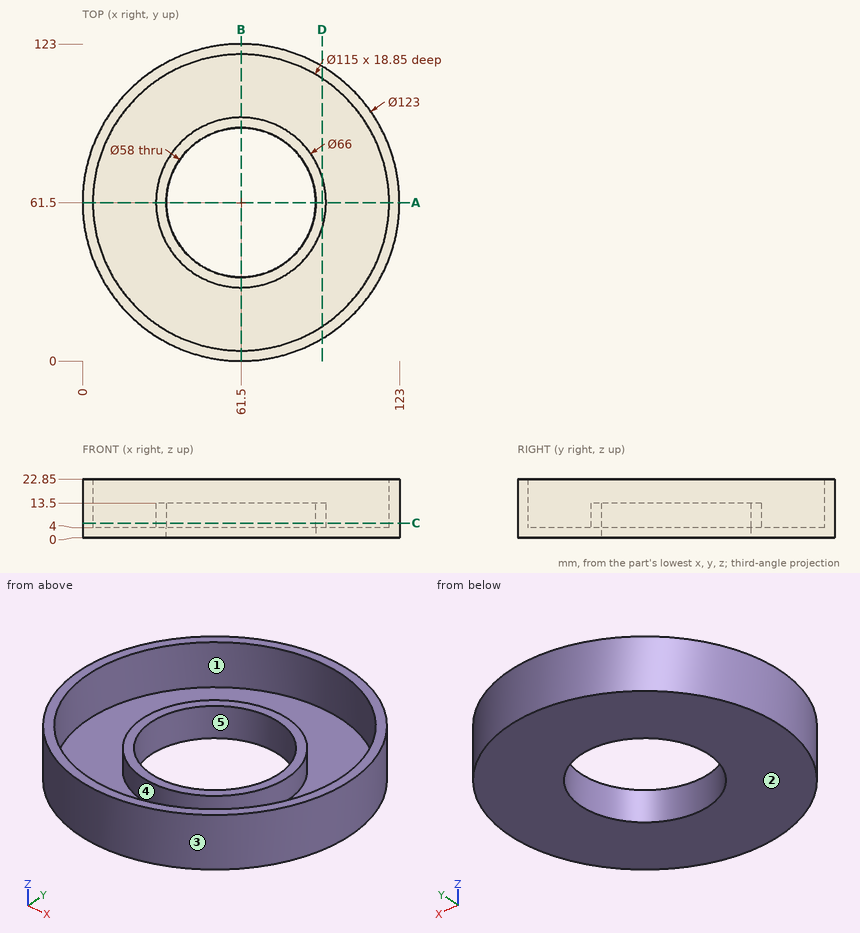
Study the drawing (mm; zero at the part's minimum x, y, z) and answer. A direction names the side the tool comes from. Coordinates: 2 decimals unless noted, no trailing zeros. Order: outer loops, then holes, each group sorted by start corner. A loop starts at its lowest first (then second) coordinate and runs counter-clockwise, first axis right, second up. Notation, with made-up numbers: M 39,68.5 L 87,68.5 A13 ccw 87,80.5 Z; hole C -21,86 d6. An arc over 180 degrees is marked long. Answer as a JSON object with one key per item and string values. Group by question number.
1. Section A-A on y = 61.5 is taken. Write down the section's boundary in (x, z), then the cut area to 3 significant figures.
2. Section D-D on x = 93 is taken. Write down the section's boundary in (y, z), then the cut area to 3 significant figures.
3. Straight lines are drawn through the part: line 1 (Y direction, x = 61.5, z = 8.5); line 2 (Y direction, x = 61.5, z = 3.5); line 3 (Y direction, x = 61.5, z = 15). For each, find the intervals that lie inside material, in ascending order.
4. A tool of negligible diameter and unlimited length cuts with its end or side. For the marked faces 4 and 5, from which of +Z, -Z, +X, -X, +Y, -Y can it reach the whole face along a straight path? Write none if from no direction.
5. Determine the mould class of the marked faces 1, 2 and 3 for opening direction X: released by +X, released by -X, zero draft, split by the parting line, or undercut.
6. Section C-C on z = 5.75 is taken. Write down the section's boundary in (x, y).
7. Flat-ended cylindrical pins translate along their axes: P1, Ø5, axis at x = 97.5, y = 74.5, coming from the +Z side; P2, Ø10, axis at y = 98.5, z = 4.5, coming from the +X side; P3, Ø10, axis at x = 98, z = 5.5, coming from the +Y side. Find the tip coordinate at first contact, or state that the pin passes through.
Values follow:
{
 "1": {"outline": "M 0,0 L 32.5,0 L 32.5,13.5 L 28.5,13.5 L 28.5,4 L 4,4 L 4,22.85 L 0,22.85 Z; M 90.5,0 L 123,0 L 123,22.85 L 119,22.85 L 119,4 L 94.5,4 L 94.5,13.5 L 90.5,13.5 Z", "area": "487 mm2"},
 "2": {"outline": "M 8.68,0 L 114.32,0 L 114.32,22.85 L 109.6,22.85 L 109.6,4 L 71.34,4 L 71.34,13.5 L 51.66,13.5 L 51.66,4 L 13.4,4 L 13.4,22.85 L 8.68,22.85 Z", "area": "787 mm2"},
 "3": {"line 1": "0 to 4, 28.5 to 32.5, 90.5 to 94.5, 119 to 123", "line 2": "0 to 32.5, 90.5 to 123", "line 3": "0 to 4, 119 to 123"},
 "4": {"face 4": "+Z", "face 5": "+Z, -Z"},
 "5": {"face 1": "undercut", "face 2": "zero draft", "face 3": "split by the parting line"},
 "6": {"outline": "C 61.5,61.5 d123; C 61.5,61.5 d66; hole C 61.5,61.5 d115; hole C 61.5,61.5 d58"},
 "7": {"P1": "z = 4", "P2": "x = 114.02", "P3": "y = 114.32"}
}
